The model under review builds one solid part; all positions refer to its coordinate system, in mm. Give positions to 0.01 mm unless a question says otherwise; leave off trailing zeros. Loops run counter-clockwise (first coordinate to the right, second up) from the corner with the lowest first, then second, coordinate; pieces in that order, holes last. Notation, with made-up numbers: M 30.25,-30 L 41.25,-30 A17 cw 41.25,1 Z; hole C 55.25,48 d10. An arc over 180 degrees is marked long. One line per item, written item: value. Start each with the question number.
Q1. To check wall thickness, follow line 1 along X through (y, z) = (0.2, 5.5); line 2 along X through (y, z) = (1.1, 8.5); line 3 along Z through (x, y) = (-32, 0.2). State the ranges of each line that lie inside material, in increasing order. Write a range as from..to.
Q2. For pin 1 (0.8 mm diameter, centred on x = -29.5, y = 0.5, fed in from +Z); pin 2 (8.5 mm diameter, centred on x = 0, z = 0, fed in from -Y), all flat-tipped, find the tip position at first contact; note any pin that passes through.
Q3. We need section C-C on z = 6. Write out the cut boundary in (x, y).
Q4. We need section B-B on y = 0.65. Give the number of separate pieces and of enclosed holes in the cut face, plus the area to 3 significant figures.
Q5. We need section A-A on x = 10. Write out the cut boundary in (y, z).
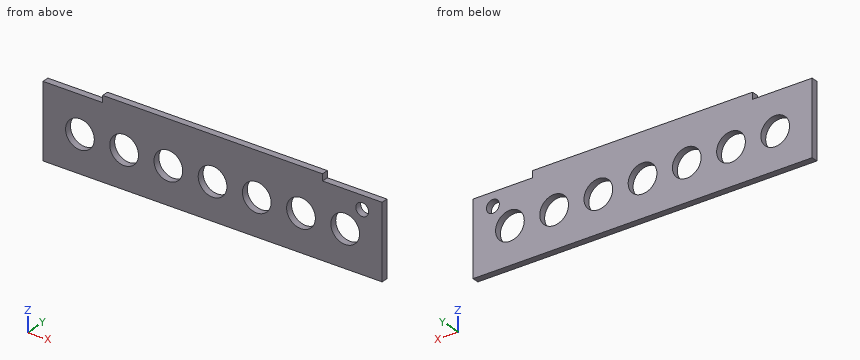
Autodesk Inventor part; units mm, degrees
ref_plane "YZ Plane" through (0, 0, 0) normal (1, 0, 0) x (0, 1, 0)
ref_plane "XZ Plane" through (0, 0, 0) normal (0, 1, 0) x (-1, 0, 0)
ref_plane "XY Plane" through (0, 0, 0) normal (0, 0, 1) x (1, 0, 0)
sketch "Sketch1" plane through (0, 0, 0) normal (0, 1, 0) x (-1, 0, 0)
  line L0 (38.35, 8.3) -> (-38.35, 8.3)
  line L1 (-38.35, 8.3) -> (-38.35, -8.3)
  line L2 (-38.35, -8.3) -> (38.35, -8.3)
  line L3 (38.35, -8.3) -> (38.35, 8.3)
  line L4 (38.35, 8.3) -> (-38.35, -8.3) construction
  line L5 (-38.35, 8.3) -> (38.35, -8.3) construction
  line L6 (24.85, 8.3) -> (-24.85, 8.3)
  line L7 (-24.85, 8.3) -> (-24.85, 9.8)
  line L8 (-24.85, 9.8) -> (24.85, 9.8)
  line L9 (24.85, 9.8) -> (24.85, 8.3)
  line L10 (-24.85, 9.8) -> (-38.35, 8.3) construction
  line L11 (24.85, 9.8) -> (38.35, 8.3) construction
  point P0 (0, 0)
  dimension "d0" = 76.7
  dimension "d1" = 16.6
  dimension "d16" = 1.5
  dimension "d17" = 13.5
extrude "Extrusion1" add sketch "Sketch1" along normal blind 1.5
sketch "Sketch2" plane through (0, 0, 0) normal (0, 1, 0) x (-1, 0, 0)
  circle A0 centre (30, 0) radius 3.25
  line L0 (30, 0) -> (0, 0) construction
  dimension "d4" = 6.5
  dimension "d5" = 30
extrude "Extrusion2" cut sketch "Sketch2" along normal through all
pattern_linear "Rectangular Pattern1" count 7 spacing 10 along (1, 0, 0) of "Extrusion2"
sketch "Sketch3" plane through (0, 0, 0) normal (0, 1, 0) x (-1, 0, 0)
  circle A0 centre (-33.85, 5.3) radius 1.45
  line L0 (38.35, -8.3) -> (38.35, 8.3) construction
  line L1 (-33.85, 5.3) -> (-33.85, 8.3) construction
  line L2 (38.35, 8.3) -> (-38.35, 8.3) construction
  line L3 (-33.85, 5.3) -> (-38.35, 5.3) construction
  line L4 (-38.35, 8.3) -> (-38.35, -8.3) construction
  point P0 (0, 0)
  dimension "d11" = 2.9
  dimension "d12" = 3
  dimension "d18" = 4.5
extrude "Extrusion3" cut sketch "Sketch3" along normal through all
properties part number "teensy_led_lid"
Solved:
1. line 1: -38.35..32.41, 35.29..38.35
1. line 2: -24.85..24.85
1. line 3: -8.3..-2.56, 2.56..8.3
2. pin 1: z = 8.3
2. pin 2: y = 0
3. outline: M -38.35,0 L 32.58,0 L 32.58,1.5 L -38.35,1.5 Z; M 35.12,0 L 38.35,0 L 38.35,1.5 L 35.12,1.5 Z
4. separate pieces: 1
4. enclosed holes: 8
4. area: 1,110 mm2
5. outline: M 0,-8.3 L 1.5,-8.3 L 1.5,-3.25 L 0,-3.25 Z; M 0,3.25 L 1.5,3.25 L 1.5,9.8 L 0,9.8 Z
